```python
from build123d import *

# Parameters (mm, degrees)
BASE_DEPTH              = 3
BASE_DEPTH_BACK         = 6
SKETCH1_R               = 10
SKETCH3_R               = 1.6
HOLE2_DEPTH             = 19.1581212
HOLE2MIRROR_COUNT       = 2
SKETCH4_R               = 1.6
HOLE3_DEPTH             = 19.100993715
SKETCH5_R               = 1.6
CUT_EXTRUDE1_DEPTH      = 19.311666101
SKETCH6_R               = 1.6
CUT_EXTRUDE2_DEPTH      = 19.560472272
SKETCH7_R               = 1.6
CUT_EXTRUDE3_DEPTH      = 19.646604846
FILLET1_R               = 2
CUT_EXTRUDE_THIN1_DEPTH = 1


with BuildPart() as part:
    # Sketch1 → base (new, two sides: drawn at the far end of the back side and taken through both)
    with BuildSketch(Plane(origin=(0, 0, 0), x_dir=(1, 0, 0), z_dir=(0, 1, 0)).offset(-BASE_DEPTH_BACK)):
        with Locations(Location((0, 0, 0), (0, 0, 270))):
            Circle(SKETCH1_R)
    extrude(amount=BASE_DEPTH + BASE_DEPTH_BACK)

    # Sketch3 → hole2 (cut, through all)
    with BuildSketch(Plane(origin=(-0.941672921, -1.236067977, 3.685836142), x_dir=(-0.9718935871364875, 0.07382318789513377, -0.22354639834264944), z_dir=(0.23541823021467095, 0.3090169943749464, -0.921459035481267))):
        with Locations(Location((0, 0, 0), (0, 0, 90.062171088))):
            Circle(SKETCH3_R)
    hole2 = extrude(amount=-HOLE2_DEPTH, mode=Mode.SUBTRACT)

    # hole2mirror: hole2 ×2 about axis
    hole2mirror_axis = Axis((0, 5.5, 0), (0, -1, 0))
    for i in range(1, HOLE2MIRROR_COUNT):
        add(hole2.rotate(hole2mirror_axis, i * 360 / HOLE2MIRROR_COUNT), mode=Mode.SUBTRACT)

    # Sketch4 → hole3 (cut, through all)
    with BuildSketch(Plane(origin=(-3.717841, -1.236067977, 0.806098168), x_dir=(-0.19123247894507908, -0.06357892752956036, -0.979483465389136), z_dir=(0.9294602499075393, 0.30901699437494623, -0.20152454200243008))):
        with Locations(Location((0, 0, 0), (0, 0, 90))):
            Circle(SKETCH4_R)
    extrude(amount=-HOLE3_DEPTH, mode=Mode.SUBTRACT)

    # Sketch5 → Cut-Extrude1 (cut, through all)
    with BuildSketch(Plane(origin=(3.671965021, -1.093066116, -1.149730122), x_dir=(0.2754858058396647, -0.08200628219437099, 0.9578008876909271), z_dir=(-0.9179912552075574, 0.27326652891267317, 0.2874325304110031))):
        with Locations(Location((0, 0, 0), (0, 0, 4.890463))):
            Circle(SKETCH5_R)
    extrude(amount=-CUT_EXTRUDE1_DEPTH, mode=Mode.SUBTRACT)

    # Sketch6 → Cut-Extrude2 (cut, through all)
    with BuildSketch(Plane(origin=(2.875583134, -1.236067977, 2.490613899), x_dir=(-0.5720437997755544, 0.24589274231852376, 0.782497699941298), z_dir=(-0.7188957835464718, 0.30901699437494723, -0.6226534747245682))):
        with Locations(Location((0, 0, 0), (0, 0, 345.016140445))):
            Circle(SKETCH6_R)
    extrude(amount=-CUT_EXTRUDE2_DEPTH, mode=Mode.SUBTRACT)

    # Sketch7 → Cut-Extrude3 (cut, through all)
    with BuildSketch(Plane(origin=(-2.670502563, -1.093066116, -2.770130417), x_dir=(0.7444971483747472, -0.2450509606833859, -0.6210265877802813), z_dir=(0.6676256406564008, 0.2732665289126714, 0.6925326043690294))):
        with Locations(Location((0, 0, 0), (0, 0, 14.758597305))):
            Circle(SKETCH7_R)
    extrude(amount=-CUT_EXTRUDE3_DEPTH, mode=Mode.SUBTRACT)

    # Fillet1
    fillet1_edges = [part.edges().sort_by_distance(p)[0] for p in [
        (0, 3, -10),
    ]]
    fillet(fillet1_edges, radius=FILLET1_R)

    # Sketch9 → Cut-Extrude-Thin1 (cut)
    with BuildSketch(Plane(origin=(0, 3, 0), x_dir=(1, 0, 0), z_dir=(0, 1, 0))):
        Polygon((-4.40005736, 3.518760981), (-0.246688962, -1.237871846), (6.097894842, 1.902273668), (5.210740629, 3.694746095), (0.246688962, 1.237871846), (-2.893541545, 4.834211512), align=None)
    extrude(amount=-CUT_EXTRUDE_THIN1_DEPTH, mode=Mode.SUBTRACT)


solid = part.part
```
Work out the finished part from the listing and answer in its coordinate system (mm). A direction names the side the tool comes from. Give positions to 0.01 mm unless a question says otherwise; leave off trailing zeros. Loops run counter-clockwise (first coordinate to the right, second up) from the corner with the lowest first, then second, coordinate; pieces in that order, holes last. Notation, with made-up numbers: (72, 56.25) -> (126, 56.25) arc R16 ccw to (126, 64.25) -> close; hole circle Ø2 at (1.5, 60.5). An arc over 180 degrees is marked (long way). Write item = value, one per line. Start each with the question number.
(1) Which of the six approach directions +Z, -Z, +X, -X, +Y, -Y give full straight-line access (tool end or side, diameter ignored) to faces 1 (the flat face through (2.88, 2.51, -0.31)), 2 (the flat face through (3.671, -1.072, -1.173)), 3 (the flat face through (0, 3, 2))?
(2) Given pin 1 Ø1 at (x, y) = (6.5, -4) entering from +Z; pin 2 Ø1 at (x, z) = (-7, 5.5) entering from +Y; pin 3 Ø3 at (y, z) = (1.5, 2) entering from -X, each flat-ended and moving along its own axis, determine where each tip first touches the part or whether it passes through.
(3) Find section A-A on y = 2.5. Give the vertices of the cut face in (x, z).
(4) Find the intervals of material crossed by probe 1 along Z at (x, y) = (4.25, -2.75); probe 2 along Z at (x, y) = (6.5, -1.75); probe 3 along Y at (x, z) = (-3, 7.5), in increasing order. Write a range as from..to.
(5) The mould has two halves that part along Z. Classify faces 4 (the cylindrical face through (6.26, -3.52, -2.32)), 5 (the flat face through (0, -6, 0)), 6 (the cylindrical face through (6.76, -2.55, -7.37)): +Z half, -Z half, draft (parallel to the pull), parting line (faces both ways), or undercut.
(6) Find section B-B on z = 0. Give the number of separate pieces and of enclosed holes in the cut face, and give its area (3 significant figures).
From the geometry:
q1.face_1 = +Y
q1.face_2 = none
q1.face_3 = +Z, -Z, +X, -X, +Y
q2.pin_1 = 8
q2.pin_2 = 2.96
q2.pin_3 = -9.98
q3.outline = circle Ø18.65 at (0, 0); hole (-4.4, -3.52) -> (-2.89, -4.83) -> (0.25, -1.24) -> (5.21, -3.69) -> (6.1, -1.9) -> (-0.25, 1.24) -> close
q4.probe_1 = -9.05..-2.22, -0.69..2.24, 5.7..9.05
q4.probe_2 = -7.6..-3.68, -0.36..3.67, 6.94..7.6
q4.probe_3 = -6..-3.87, -1.33..3
q5.face_4 = undercut
q5.face_5 = draft
q5.face_6 = parting line
q6.separate_pieces = 1
q6.enclosed_holes = 2
q6.area = 165 mm^2
